Geometry: final body of the model. Coordinates: model frame, mm. Face numbers are marked on the shaded views. A direction names the side the tool comes from. Coordinates: 2 decimals unless noted, no trailing zeros. Order: outer loops, then holes, each group sorted by start corner. A loop starts at its lowest first (then second) coordinate and runs counter-clockwise, first axis right, second up. Notation, with made-up numbers: (49, 78) - (91, 78) arc R19 cw to (91, 95) - close; hole circle Ø6 at (80, -11.5). An arc over 180 degrees is marked (long way). Use one line per item in the form item = value. Start each with the question number.
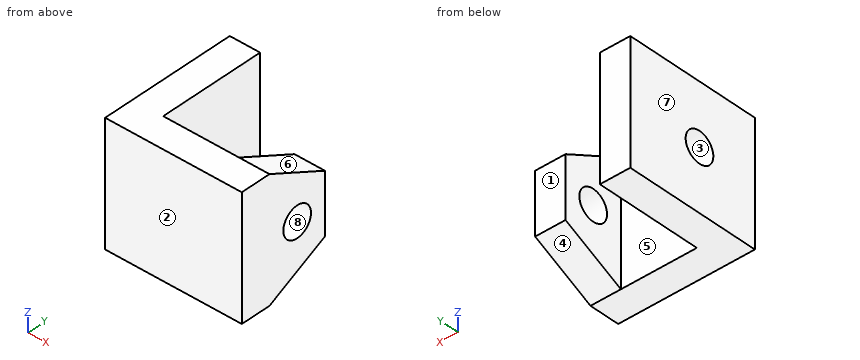
```python
from build123d import *

# Parameters (mm, degrees)
EXTRUDE_1_DEPTH          = 20
SKETCH_1_3_W             = 10
SKETCH_1_3_H             = 20
EXTRUDE_2_DEPTH          = 20
SKETCH_2_R               = 5
CUT_EXTRUDE_1_DEPTH      = 10
CUT_EXTRUDE_2_DEPTH      = 67.708320321
CUT_EXTRUDE_2_DEPTH_BACK = 10
CUT_EXTRUDE_3_DEPTH      = 67.708320321
CUT_EXTRUDE_3_DEPTH_BACK = 10
CUT_EXTRUDE_START        = -10
SKETCH_9_R               = 5
CUT_EXTRUDE_4_DEPTH      = 10


with BuildPart() as part:
    # Sketch 1 → Extrude 1 (new, symmetric)
    with BuildSketch(Plane.XY):
        Polygon((10, 45), (0, 45), (0, 0), (45, 0), (45, 10), (10, 10), align=None)
    extrude(amount=EXTRUDE_1_DEPTH, both=True)

    # Sketch 1_3 → Extrude 2 (add, symmetric)
    with BuildSketch(Plane.XY):
        with Locations((40, 20)):
            Rectangle(SKETCH_1_3_W, SKETCH_1_3_H)
    extrude(amount=EXTRUDE_2_DEPTH, both=True)

    # Sketch 2 → Cut-Extrude 1 (cut)
    with BuildSketch(Plane(origin=(45, 0, 0), x_dir=(0, 0, -1), z_dir=(1, 0, 0))):
        with Locations((0, 20)):
            Circle(SKETCH_2_R)
    extrude(amount=-CUT_EXTRUDE_1_DEPTH, mode=Mode.SUBTRACT)

    # Sketch 2_5 → Cut-Extrude 2 (cut, two sides: drawn at the far end of the back side and taken through both)
    with BuildSketch(Plane(origin=(45, 0, 0), x_dir=(0, 0, -1), z_dir=(1, 0, 0)).offset(-CUT_EXTRUDE_2_DEPTH_BACK)):
        Polygon((-20, 10), (-10, 30), (-20, 30), align=None)
    extrude(amount=CUT_EXTRUDE_2_DEPTH + CUT_EXTRUDE_2_DEPTH_BACK, mode=Mode.SUBTRACT)

    # Sketch 7 → Cut-Extrude 3 (cut, two sides: drawn at the far end of the back side and taken through both)
    with BuildSketch(Plane(origin=(45, 0, 0), x_dir=(0, 0, -1), z_dir=(1, 0, 0)).offset(-CUT_EXTRUDE_3_DEPTH_BACK)):
        Polygon((20, 30), (10, 30), (20, 10), align=None)
    extrude(amount=CUT_EXTRUDE_3_DEPTH + CUT_EXTRUDE_3_DEPTH_BACK, mode=Mode.SUBTRACT)

    # Sketch 9 → Cut-Extrude 4 (cut)
    with BuildSketch(Plane.ZY.offset(CUT_EXTRUDE_START)):
        with Locations(Location((0, 20, 0), (0, 0, 180))):
            Circle(SKETCH_9_R)
    extrude(amount=CUT_EXTRUDE_4_DEPTH, mode=Mode.SUBTRACT)


solid = part.part
```
(1) Cut plane A-A on y = 17. Return the cut outline in (x, z).
(2) Cut plane C-C on z = 0. Return the cut outline in (x, y), plus the area to 3 significant figures.
(3) Set-up query: the marked faces 1, 2, 3, 4 and 5. Return all of +Z, -Z, +X, -X, +Y, -Y with unobstructed straight access to the full face (end or side cutting, diameter ignored); none if empty.
(4) Cut plane B-B on x = 40.5. Return the cut outline in (y, z), plus the area to 3 significant figures.
(5) Material intervals for L1, parallel to X at y = 26, z = -4.5; L2, parallel to Y at x = 7, z = 0; L3, parallel to Y at x = 39.75, z = 0, sorted ascending. Write a range as from..to.
(6) Contact query for flat-ended pins moving along their axis: pin 1 Ø1.5 at (x, z) = (40, 13.5) entering from +Y; pin 2 Ø3 at (x, y) = (35, 25.5) entering from +Z; pin 3 Ø12 at (x, z) = (25.5, 3) entering from +Y; pin 4 Ø8 at (y, z) = (20, 0) entering from -X. Output: stop coordinate, or through.
(7) Cut plane D-D on z = 17.5. Return the cut outline in (x, y), plus the area to 3 significant figures.
(8) Draft query along Y for the marked faces 6, 7 and 8. Return one class per face: released by +Y, released by -Y, zero draft, split by the parting line, or undercut.
Check sheet entries:
q1.outline = (0, -20) - (10, -20) - (10, -4) - (0, -4) - close; (0, 4) - (10, 4) - (10, 20) - (0, 20) - close; (35, -16.5) - (45, -16.5) - (45, -4) - (35, -4) - close; (35, 4) - (45, 4) - (45, 16.5) - (35, 16.5) - close
q2.outline = (0, 0) - (45, 0) - (45, 15) - (35, 15) - (35, 10) - (10, 10) - (10, 15) - (0, 15) - close; (0, 25) - (10, 25) - (10, 45) - (0, 45) - close; (35, 25) - (45, 25) - (45, 30) - (35, 30) - close
q2.area = 800 mm^2
q3.face_1 = +Z, -Z, +X, +Y
q3.face_2 = +Z, -Z, +X, -X, -Y
q3.face_3 = +X, -X
q3.face_4 = -Z, +X, +Y
q3.face_5 = +Z, -Z, +Y
q4.outline = (0, -20) - (10, -20) - (30, -10) - (30, 10) - (10, 20) - (0, 20) - close; hole circle Ø10 at (20, 0)
q4.area = 921 mm^2
q5.L1 = 0..10, 35..45
q5.L2 = 0..15, 25..45
q5.L3 = 0..15, 25..30
q6.pin_1 = 24.5
q6.pin_2 = 13
q6.pin_3 = 10
q6.pin_4 = through
q7.outline = (0, 0) - (45, 0) - (45, 15) - (35, 15) - (35, 10) - (10, 10) - (10, 45) - (0, 45) - close
q7.area = 850 mm^2
q8.face_6 = released by +Y
q8.face_7 = zero draft
q8.face_8 = undercut
